Autodesk Inventor part; units mm, degrees
ref_plane "YZ Plane" through (0, 0, 0) normal (1, 0, 0) x (0, 1, 0)
ref_plane "XZ Plane" through (0, 0, 0) normal (0, 1, 0) x (-1, 0, 0)
ref_plane "XY Plane" through (0, 0, 0) normal (0, 0, 1) x (1, 0, 0)
sketch "Sketch1" plane through (0, 0, 0) normal (1, 0, 0) x (0, 1, 0)
  line L0 (6.35, 0) -> (69.85, 0)
  line L1 (76.2, -6.35) -> (76.2, -120.65)
  line L2 (69.85, -127) -> (6.35, -127)
  line L3 (0, -120.65) -> (0, -6.35)
  arc A0 (76.2, -6.35) -> (69.85, 0) centre (69.85, -6.35) ccw
  arc A1 (69.85, -127) -> (76.2, -120.65) centre (69.85, -120.65) ccw
  arc A2 (0, -120.65) -> (6.35, -127) centre (6.35, -120.65) ccw
  arc A3 (6.35, 0) -> (0, -6.35) centre (6.35, -6.35) ccw
  line L4 (69.85, -120.65) -> (69.85, -6.35)
  line L5 (69.85, -6.35) -> (6.35, -6.35)
  line L6 (6.35, -6.35) -> (6.35, -120.65)
  line L7 (6.35, -120.65) -> (69.85, -120.65)
  point P0 (0, 0)
  point P1 (76.2, -127)
  point P2 (76.2, 0)
  point P3 (0, -127)
  dimension "d0" = 76.2
  dimension "d1" = 127
  dimension "d2" = 6.35
  dimension "d3" = 6.35
  dimension "d4" = 6.35
extrude "Extrusion1" add sketch "Sketch1" against normal blind 101.6
sketch "Sketch2" plane through (0, 76.2, -6.35) normal (0, 1, 0) x (1, 0, 0)
  line L0 (0, 0) -> (0, 114.3) construction
  line L1 (0, 57.15) -> (-101.6, 57.15) construction
  line L2 (-101.6, 114.3) -> (-101.6, 0) construction
  line L3 (0, 83.65) -> (-45.4, 83.65) construction
  line L4 (-45.4, 83.65) -> (-45.4, 110.65) construction
  line L5 (-45.4, 110.65) -> (0, 110.65) construction
  line L6 (0, 110.65) -> (0, 83.65) construction
  line L7 (-32.7, 107.15) -> (-12.7, 107.15) construction
  line L8 (-12.7, 107.15) -> (-12.7, 87.15) construction
  line L9 (-12.7, 87.15) -> (-32.7, 87.15) construction
  line L10 (-32.7, 87.15) -> (-32.7, 107.15) construction
  line L11 (-32.7, 107.15) -> (-32.7, 110.65) construction
  line L12 (-32.7, 107.15) -> (-45.4, 107.15) construction
  line L13 (-12.7, 87.15) -> (-12.7, 83.65) construction
  line L14 (-12.7, 87.15) -> (0, 87.15) construction
  circle A0 centre (-32.7, 107.15) radius 1.6
  circle A1 centre (-12.7, 107.15) radius 1.6
  circle A2 centre (-12.7, 87.15) radius 1.6
  circle A3 centre (-32.7, 87.15) radius 1.6
  line L15 (0, 114.3) -> (0, 0) construction
  line L16 (-50.8, 57.15) -> (-50.8, 128.3257) construction
  line L17 (-101.6, 83.65) -> (-56.2, 83.65) construction
  line L18 (-56.2, 83.65) -> (-56.2, 110.65) construction
  line L19 (-56.2, 110.65) -> (-101.6, 110.65) construction
  line L20 (-101.6, 110.65) -> (-101.6, 83.65) construction
  line L21 (-68.9, 107.15) -> (-88.9, 107.15) construction
  line L22 (-88.9, 107.15) -> (-88.9, 87.15) construction
  line L23 (-88.9, 87.15) -> (-68.9, 87.15) construction
  line L24 (-68.9, 87.15) -> (-68.9, 107.15) construction
  line L25 (-68.9, 107.15) -> (-68.9, 110.65) construction
  line L26 (-68.9, 107.15) -> (-56.2, 107.15) construction
  line L27 (-88.9, 87.15) -> (-88.9, 83.65) construction
  line L28 (-88.9, 87.15) -> (-101.6, 87.15) construction
  circle A4 centre (-68.9, 107.15) radius 1.6
  circle A5 centre (-88.9, 107.15) radius 1.6
  circle A6 centre (-88.9, 87.15) radius 1.6
  circle A7 centre (-68.9, 87.15) radius 1.6
  line L29 (0, 30.65) -> (-45.4, 30.65) construction
  line L30 (-45.4, 30.65) -> (-45.4, 3.65) construction
  line L31 (-45.4, 3.65) -> (0, 3.65) construction
  line L32 (0, 3.65) -> (0, 30.65) construction
  line L33 (-32.7, 7.15) -> (-12.7, 7.15) construction
  line L34 (-12.7, 7.15) -> (-12.7, 27.15) construction
  line L35 (-12.7, 27.15) -> (-32.7, 27.15) construction
  line L36 (-32.7, 27.15) -> (-32.7, 7.15) construction
  line L37 (-32.7, 7.15) -> (-32.7, 3.65) construction
  line L38 (-32.7, 7.15) -> (-45.4, 7.15) construction
  line L39 (-12.7, 27.15) -> (-12.7, 30.65) construction
  line L40 (-12.7, 27.15) -> (0, 27.15) construction
  circle A8 centre (-32.7, 7.15) radius 1.6
  circle A9 centre (-12.7, 7.15) radius 1.6
  circle A10 centre (-12.7, 27.15) radius 1.6
  circle A11 centre (-32.7, 27.15) radius 1.6
  line L41 (-68.9, 7.15) -> (-88.9, 7.15) construction
  line L42 (-88.9, 27.15) -> (-68.9, 27.15) construction
  line L43 (-88.9, 27.15) -> (-88.9, 30.65) construction
  line L44 (-88.9, 7.15) -> (-88.9, 27.15) construction
  circle A12 centre (-88.9, 27.15) radius 1.6
  circle A13 centre (-88.9, 7.15) radius 1.6
  line L45 (-101.6, 30.65) -> (-56.2, 30.65) construction
  line L46 (-101.6, 3.65) -> (-101.6, 30.65) construction
  line L47 (-88.9, 27.15) -> (-101.6, 27.15) construction
  line L48 (-56.2, 3.65) -> (-101.6, 3.65) construction
  line L49 (-68.9, 27.15) -> (-68.9, 7.15) construction
  line L50 (-68.9, 7.15) -> (-68.9, 3.65) construction
  circle A14 centre (-68.9, 7.15) radius 1.6
  circle A15 centre (-68.9, 27.15) radius 1.6
  line L51 (-56.2, 30.65) -> (-56.2, 3.65) construction
  line L52 (-68.9, 7.15) -> (-56.2, 7.15) construction
  point P0 (0, -6.35)
  dimension "d7" = 45.4
  dimension "d8" = 27
  dimension "d9" = 20
  dimension "d10" = 20
  dimension "d11" = 3.2
  dimension "d12" = 3.2
  dimension "d13" = 3.2
  dimension "d14" = 3.2
  dimension "d15" = 100
extrude "Extrusion2" cut sketch "Sketch2" against normal up to next
sketch "Sketch3" plane through (0, 6.35, -127) normal (0, 0, -1) x (-1, 0, 0)
  line L0 (38.3, 37.65) -> (63.3, 37.65) construction
  line L1 (63.3, 37.65) -> (63.3, 12.65) construction
  line L2 (63.3, 12.65) -> (38.3, 12.65) construction
  line L3 (38.3, 12.65) -> (38.3, 37.65) construction
  circle A0 centre (38.3, 37.65) radius 2.1
  circle A1 centre (63.3, 37.65) radius 2.1
  circle A2 centre (63.3, 12.65) radius 2.1
  circle A3 centre (38.3, 12.65) radius 2.1
  line L4 (0, -6.35) -> (101.6, -6.35) construction
  line L5 (38.3, 25.15) -> (0, 25.15) construction
  line L6 (0, 0) -> (0, 63.5) construction
  line L7 (63.3, 25.15) -> (101.6, 25.15) construction
  line L8 (101.6, 63.5) -> (101.6, 0) construction
  dimension "d18" = 25
  dimension "d19" = 25
  dimension "d20" = 4.2
  dimension "d21" = 4.2
  dimension "d22" = 4.2
  dimension "d23" = 4.2
  dimension "d24" = 19
extrude "Extrusion3" cut sketch "Sketch3" against normal up to next
equation "\"d12\" = d11"
equation "\"d13\" = d11"
equation "\"d14\" = d11"
equation "\"d16\" = d12"
equation "\"d21\" = d20"
equation "\"d22\" = d20"
equation "\"d23\" = d20"
properties part number "3in x 5in Steel Rectangular Tubing 4in long"
Verification items for the finished model (mm, model axes). A direction names the side the tool comes from. Coordinates: 2 decimals unless noted, no trailing zeros. Order: outer loops, then holes, each group sorted by start corner. A loop starts at its lowest first (then second) coordinate and runs counter-clockwise, first axis right, second up. Notation, with made-up numbers: M 85,83 L 104,83 A19 cw 104,107 Z; hole C -5.5,32.25 d5. An arc over 180 degrees is marked long. One line per item, written item: value. Start each with the question number.
Item 1: Mould release check, pull along X, two halves, no side actions. Record for faces 5 (the flat face through (0, 4, -63)), 6 (the cylindrical face through (-87.374, 73.069, -93.981)), 7 (the flat face through (-101.6, 4, -63)): released by +X, released by -X, zero draft, split by the parting line, or undercut.
Item 2: Sectioned sample at B-B (z = -79.5). Enter the section's corners in (x, y), then the cut area to 3 significant figures.
Item 3: Scan lines: probe 1 along X at (y, z) = (74.25, -113.5); probe 2 along Y at (x, z) = (-77.5, -46.5); probe 3 along Z at (x, y) = (-91, 56.5). Record each from-to range of solid material in increasing order.
Item 4: Access from +Z, -Z, +X, -X, +Y, -Y to the whole of each face (thin tool, end or side, straight path). Record for faces 1 (the cylindrical face through (-31.174, 73.069, -93.981)), 2 (the cylindrical face through (-50.09, 74.29, -125.19)), 3 (the cylindrical face through (-36.2, 19.09, -123.87)), 4 (the flat face through (-50, 39, -6.35)).
Item 5: Sectioned sample at D-D (z = -13.5). Enter the section's corners in (x, y).
Item 6: Sectioned sample at C-C (y = 48.5). Enter the section's corners in (x, z).
Item 7: Gauge pin test, flat ends, axial feed: pin 1 (4 mm diameter, centred on x = -63.3, y = 44, fed in from -Z); pin 2 (3 mm diameter, centred on x = -12.7, z = -113.5, fed in from +Y). Record the tip position at first contact, or that the pin passes through.
Item 8: Sectioned sample at A-A (x = -88.9). Enter the section's corners in (y, z).
Conclusion:
1. face 5: released by +X
1. face 6: undercut
1. face 7: released by -X
2. outline: M -101.6,0 L 0,0 L 0,6.35 L -101.6,6.35 Z; M -101.6,69.85 L 0,69.85 L 0,76.2 L -101.6,76.2 Z
2. area: 1,290 mm^2
3. probe 1: x = -101.6 to -90.5, -87.3 to -70.5, -67.3 to -34.3, -31.1 to -14.3, -11.1 to 0
3. probe 2: y = 0 to 6.35, 69.85 to 76.2
3. probe 3: z = -127 to -120.65, -6.35 to 0
4. face 1: +Y
4. face 2: -Z, +X, -X, +Y
4. face 3: -Z
4. face 4: +X, -X
5. outline: M -101.6,0 L 0,0 L 0,6.35 L -101.6,6.35 Z; M -101.6,69.85 L -90.5,69.85 L -90.5,76.2 L -101.6,76.2 Z; M -87.3,69.85 L -70.5,69.85 L -70.5,76.2 L -87.3,76.2 Z; M -67.3,69.85 L -34.3,69.85 L -34.3,76.2 L -67.3,76.2 Z; M -31.1,69.85 L -14.3,69.85 L -14.3,76.2 L -31.1,76.2 Z; M -11.1,69.85 L 0,69.85 L 0,76.2 L -11.1,76.2 Z
6. outline: M -101.6,-127 L 0,-127 L 0,-120.65 L -101.6,-120.65 Z; M -101.6,-6.35 L 0,-6.35 L 0,0 L -101.6,0 Z
7. pin 1: stops at z = -6.35
7. pin 2: stops at y = 6.35
8. outline: M 0,-120.65 A6.35 ccw 6.35,-127 L 69.85,-127 A6.35 ccw 76.2,-120.65 L 76.2,-115.1 L 69.85,-115.1 L 69.85,-120.65 L 6.35,-120.65 L 6.35,-6.35 L 69.85,-6.35 L 69.85,-11.9 L 76.2,-11.9 L 76.2,-6.35 A6.35 ccw 69.85,0 L 6.35,0 A6.35 ccw 0,-6.35 Z; M 69.85,-111.9 L 76.2,-111.9 L 76.2,-95.1 L 69.85,-95.1 Z; M 69.85,-91.9 L 76.2,-91.9 L 76.2,-35.1 L 69.85,-35.1 Z; M 69.85,-31.9 L 76.2,-31.9 L 76.2,-15.1 L 69.85,-15.1 Z
